The model under review builds one solid part; all positions refer to its coordinate system, in mm. Face numbers are marked on the shaded views. Coordinates: 2 decimals unless noted, no trailing zeros. Write each loop counter-clockwise with the first axis right and the second up, starting at its lowest first coordinate (ties: lowest second). Pieces come first, ordered by that corner, then holes. Notation, with made-up numbers: M 18,-15.5 L 71,-15.5 A29 cw 71,14.5 Z; hole C 82,31.25 d8. An arc over 180 degrees is marked long. Answer as a JSON object with one key per item and string values.
```python
from build123d import *

# Parameters (mm, degrees)
SKETCH1_W           = 24.5
SKETCH1_H           = 24.5
BOSS_EXTRUDE1_DEPTH = 52.75
SKETCH3_R           = 1.3
CUT_EXTRUDE1_DEPTH  = 10
SKETCH4_W           = 1.9
SKETCH4_H           = 1.9
CUT_EXTRUDE2_DEPTH  = 0.2
FILLET1_R           = 5
CUT_EXTRUDE3_START  = -4
CUT_EXTRUDE3_DEPTH  = 2.5
SKETCH6_R           = 2.5
CUT_EXTRUDE4_DEPTH  = 7


with BuildPart() as part:
    # Sketch1 → Boss-Extrude1 (new body)
    with BuildSketch(Plane(origin=(0, 0, 0), x_dir=(1, 0, 0), z_dir=(0, 1, 0))):
        Rectangle(SKETCH1_W, SKETCH1_H)
    extrude(amount=BOSS_EXTRUDE1_DEPTH)

    # Sketch3 → Cut-Extrude1 (cut)
    with BuildSketch(Plane.XZ):
        with Locations((-7.5, 0)):
            Circle(SKETCH3_R)
        with Locations((7.5, 0)):
            Circle(SKETCH3_R)
    extrude(amount=-CUT_EXTRUDE1_DEPTH, mode=Mode.SUBTRACT)

    # Sketch4 → Cut-Extrude2 (cut)
    with BuildSketch(Plane(origin=(0, 52.75, 0), x_dir=(1, 0, 0), z_dir=(0, 1, 0))):
        Polygon((0.95, 12.25), (0.95, 5.05), (-0.95, 5.05), (-0.95, 12.25), (-5.05, 12.25), (-5.05, 5.05), (-12.25, 5.05), (-12.25, 0.95), (-5.05, 0.95), (-5.05, -0.95), (-12.25, -0.95), (-12.25, -5.05), (-5.05, -5.05), (-5.05, -12.25), (-0.95, -12.25), (-0.95, -5.05), (0.95, -5.05), (0.95, -12.25), (5.05, -12.25), (5.05, -5.05), (12.25, -5.05), (12.25, -0.95), (5.05, -0.95), (5.05, 0.95), (12.25, 0.95), (12.25, 5.05), (5.05, 5.05), (5.05, 12.25), align=None)
        Rectangle(SKETCH4_W, SKETCH4_H, mode=Mode.SUBTRACT)
    extrude(amount=-CUT_EXTRUDE2_DEPTH, mode=Mode.SUBTRACT)

    # Fillet1
    fillet1_edges = [part.edges().sort_by_distance(p)[0] for p in [
        (12.25, 26.375, 12.25),
        (-12.25, 26.375, 12.25),
        (-12.25, 26.375, -12.25),
        (12.25, 26.375, -12.25),
    ]]
    fillet(fillet1_edges, radius=FILLET1_R)

    # Sketch5 → Cut-Extrude3 (cut)
    with BuildSketch(Plane.XZ.offset(CUT_EXTRUDE3_START)):
        Polygon((-9.08771324, -2.75), (-5.91228676, -2.75), (-4.324573519, 0), (-5.91228676, 2.75), (-9.08771324, 2.75), (-14.788950872, 2.75), (-14.788950872, -2.75), align=None)
        Polygon((9.08771324, 2.75), (5.91228676, 2.75), (4.324573519, 0), (5.91228676, -2.75), (9.08771324, -2.75), (14.28132796, -2.75), (14.28132796, 2.75), align=None)
    extrude(amount=-CUT_EXTRUDE3_DEPTH, mode=Mode.SUBTRACT)

    # Sketch6 → Cut-Extrude4 (cut)
    with BuildSketch(Plane.ZY.offset(12.25)):
        with Locations((0, 45)):
            Circle(SKETCH6_R)
    extrude(amount=-CUT_EXTRUDE4_DEPTH, mode=Mode.SUBTRACT)


solid = part.part
```
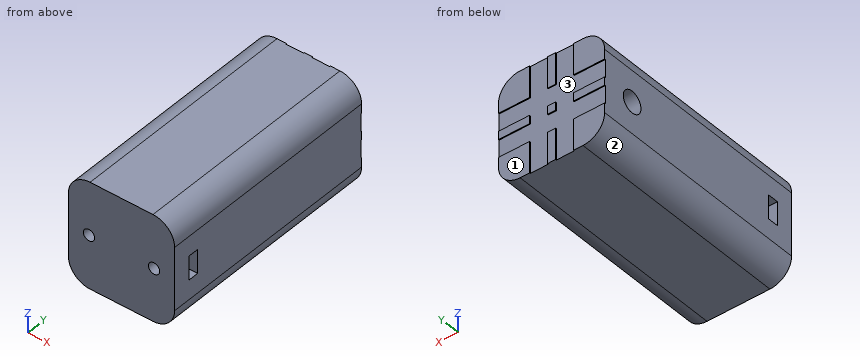
(1) Add section D-D on y = 13.5. Give the boundary of the cut face in (x, z).
Results list:
{"outline": "M -12.25,-7.25 A5 ccw -7.25,-12.25 L 7.25,-12.25 A5 ccw 12.25,-7.25 L 12.25,7.25 A5 ccw 7.25,12.25 L -7.25,12.25 A5 ccw -12.25,7.25 Z"}
(2) Wall thickness on line 1 along Y through (x, z) = (-9.5, 0); line 2 along Z through (x, y) = (7.5, 9.3); line 3 along Y through (x, z) = (-7.5, 0): over which ranges is each line inside the solid? List them lowest first. Write a range as from..to.
Results list:
{"line 1": "0..4, 6.5..42.5, 47.5..52.75", "line 2": "-12.24..-1.3, 1.3..12.24", "line 3": "10..42.5, 47.5..52.75"}
(3) Add section A-A on y = 7.5. Give the boundary of the cut face in (x, z), and give its area (3 significant figures).
Results list:
{"outline": "M -12.25,-7.25 A5 ccw -7.25,-12.25 L 7.25,-12.25 A5 ccw 12.25,-7.25 L 12.25,7.25 A5 ccw 7.25,12.25 L -7.25,12.25 A5 ccw -12.25,7.25 Z; hole C -7.5,0 d2.6; hole C 7.5,0 d2.6", "area": "568 mm²"}
(4) Add section B-B on x = -10.25. Give the boundary of the cut face in (y, z), and give its area (3 significant figures).
Results list:
{"outline": "M 0,-11.25 L 52.75,-11.25 L 52.75,-5.05 L 52.55,-5.05 L 52.55,-0.95 L 52.75,-0.95 L 52.75,0.95 L 52.55,0.95 L 52.55,5.05 L 52.75,5.05 L 52.75,11.25 L 0,11.25 Z; hole M 4,-2.75 L 6.5,-2.75 L 6.5,2.75 L 4,2.75 Z; hole C 45,0 d5", "area": "1,150 mm²"}
(5) For pin 1 Ø3 at (x, z) = (-8, 0.5) entering from -Y; pin 2 Ø1.6 at (x, z) = (-7.5, 0) entering from -Y; pin 3 Ø3 at (y, z) = (37.5, -9) entering from -X, all flat-tipped, find the tip position at first contact; note any pin that passes through.
Results list:
{"pin 1": "y = 0", "pin 2": "y = 10", "pin 3": "x = -12.24"}
(6) Add section C-C on y = 45. Give the boundary of the cut face in (x, z).
Results list:
{"outline": "M -12.25,-7.25 A5 ccw -7.25,-12.25 L 7.25,-12.25 A5 ccw 12.25,-7.25 L 12.25,7.25 A5 ccw 7.25,12.25 L -7.25,12.25 A5 ccw -12.25,7.25 L -12.25,2.5 L -5.25,2.5 L -5.25,-2.5 L -12.25,-2.5 Z"}
(7) Draft analysis for pull direction Z (two halves, no side actions). For the marked faces 1, 2 and 3, state which applies: released by +Z, released by -Z, zero draft, split by the parting line, or undercut.
Results list:
{"face 1": "zero draft", "face 2": "released by -Z", "face 3": "undercut"}
